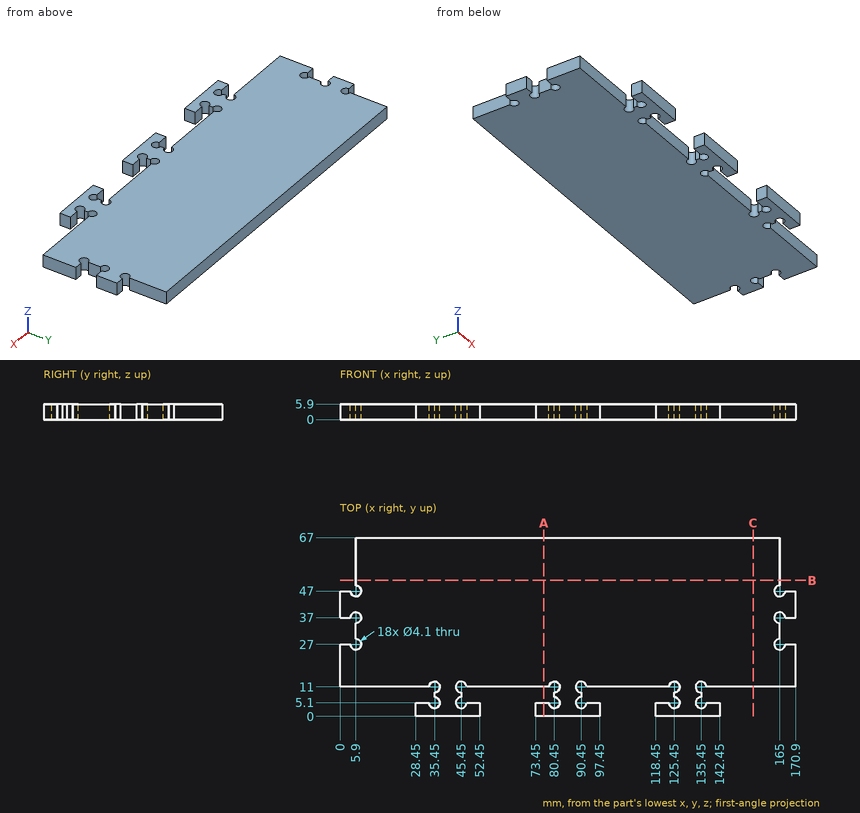
Check sheet for the drawn part. Datum: minimum x, y, z corner. Units: mm. Round coordinates to 2 decimals unless told otherwise and drop trailing zeros. Order: outer loops, then holes, each group sorted by start corner. A loop starts at its lowest first (then second) coordinate and runs counter-clockwise, first axis right, second up. Notation, with made-up numbers: (33, -16.5) - (43, -16.5) arc R28 ccw to (43, 11.5) - close; hole circle Ø11 at (-36, 14). An arc over 180 degrees is marked (long way). Use a Markdown table: item, result. Add a question column.
(1) Sectioned sample at B-B, the plane y = 51. Enter the section's corners in (x, z).
(2) Depth check by flat-ended pin: pin 1 (3 mm diameter, centred on x = 159, z = 1.5, fed in from -Y); pin 2 (1.9 mm diameter, centred on x = 169, z = 3.5, fed in from +Y); pin 3 (5.5 mm diameter, centred on x = 165, y = 37, fed in from +Z); pin 4 (1.8 mm diameter, centred on y = 31.5, z = 2, fed in from +X). Enter the tip coordinate at first touch or a pass-through.
(3) Material ranges on line 1 along Y through (x, z) = (96, 3.45); line 2 along Y through (x, z) = (105, 3.7); line 3 along Y through (x, z) = (79.5, 4.05), recorded low to high. Write a range as [from, to].
(4) Sectioned sample at C-C, the plane x = 155. Enter the section's corners in (y, z).
(5) Sectioned sample at A-A, the plane x = 76.5. Enter the section's corners in (y, z).
Answers below:
| question | item | result |
|---|---|---|
| 1 | outline | (5.9, 0) - (165, 0) - (165, 5.9) - (5.9, 5.9) - close |
| 2 | pin 1 | y = 11 |
| 2 | pin 2 | y = 47 |
| 2 | pin 3 | z = 5.9 |
| 2 | pin 4 | x = 165 |
| 3 | line 1 | [0, 5.1], [11, 67] |
| 3 | line 2 | [11, 67] |
| 3 | line 3 | [0, 3.28], [12.82, 67] |
| 4 | outline | (11, 0) - (67, 0) - (67, 5.9) - (11, 5.9) - close |
| 5 | outline | (0, 0) - (5.1, 0) - (5.1, 5.9) - (0, 5.9) - close; (11, 0) - (67, 0) - (67, 5.9) - (11, 5.9) - close |
